Autodesk Fusion 360 part; units mm, degrees
sketch "Sketch1" plane through (0, 0, 0) normal (0, 0, 1) x (1, 0, 0)
  line L0 (2.6252, 0) -> (7.4595, 0)
  line L1 (10.0424, 2.5828) -> (10.0424, 3.3)
  line L2 (0.0424, 3.3) -> (0.0424, 2.5828)
  line L3 (8.0424, 3.7) -> (8.0424, 4.8)
  line L4 (2.0424, 4.8) -> (2.0424, 3.7)
  line L5 (0.101, 2.4414) -> (2.4838, 0.0586)
  line L6 (0.0424, 2.5) -> (3.5052, 2.5) construction
  line L7 (5.0424, 3.5) -> (5.0424, 0) construction
  line L8 (9.9838, 2.4414) -> (7.601, 0.0586)
  line L9 (9.8424, 3.5) -> (8.2424, 3.5)
  line L10 (1.8424, 3.5) -> (0.2424, 3.5)
  line L11 (5.0424, 4.7) -> (5.3424, 5)
  line L12 (5.0424, 4.7) -> (6.213, 4.7) construction
  line L13 (5.0424, 4.7) -> (4.7424, 5)
  line L14 (5.0424, 4.7) -> (6.2088, 4.7) construction
  line L15 (7.8424, 5) -> (5.3424, 5)
  line L16 (4.7424, 5) -> (2.2424, 5)
  arc A0 (0.2424, 3.5) -> (0.0424, 3.3) centre (0.2424, 3.3) ccw
  arc A1 (0.0424, 2.5828) -> (0.101, 2.4414) centre (0.2424, 2.5828) ccw
  arc A2 (2.4838, 0.0586) -> (2.6252, 0) centre (2.6252, 0.2) ccw
  arc A3 (7.4595, 0) -> (7.601, 0.0586) centre (7.4595, 0.2) ccw
  arc A4 (9.9838, 2.4414) -> (10.0424, 2.5828) centre (9.8424, 2.5828) ccw
  arc A5 (10.0424, 3.3) -> (9.8424, 3.5) centre (9.8424, 3.3) ccw
  arc A6 (8.0424, 3.7) -> (8.2424, 3.5) centre (8.2424, 3.7) ccw
  arc A7 (8.0424, 4.8) -> (7.8424, 5) centre (7.8424, 4.8) ccw
  arc A8 (2.2424, 5) -> (2.0424, 4.8) centre (2.2424, 4.8) ccw
  arc A9 (1.8424, 3.5) -> (2.0424, 3.7) centre (1.8424, 3.7) ccw
  dimension "d1" = 10
  dimension "d4" = 5
  dimension "d5" = 45
  dimension "d6" = 1
  dimension "d7" = 5
  dimension "d8" = 6
  dimension "d9" = 2
  dimension "d10" = 2
  dimension "d12" = 45
  dimension "d13" = 0.3
  dimension "d14" = 5
  dimension "d15" = 1.5
  dimension "d16" = 0.2
extrude "Extrude1" add sketch "Sketch1" along normal blind 10
hole "Hole1" at (5.0424, 5, 5) direction (0, -1, 0) diameter 4.234 depth 5.834 tip angle 180 countersink diameter 6 countersink angle 90
Build history of the part. All positions in model axes, mm. A direction names the side the tool comes from. Coordinates: 2 decimals unless noted, no trailing zeros. Order: outer loops, then holes, each group sorted by start corner. A loop starts at its lowest first (then second) coordinate and runs counter-clockwise, first axis right, second up. Notation, with made-up numbers: M 69.5,36 L 117.5,36 A15 ccw 117.5,49 Z; hole C -37.75,76.5 d8. An arc over 180 degrees is marked long. One line per question, with ' | ' between items. Start each with the question number.
1. Tool access for faces 5 (the face through (7, 5, 1)), 6 (the face through (1, 3.5, 5)), 7 (the face through (8.042, 4, 5)): list every direction of +Z, -Z, +X, -X, +Y, -Y with a clear straight run to the whole face (end or side of a thin tool).
2. Flat gauge pins, fed straight in: P1, Ø1, axis at x = 5, z = 6.5, coming from the +Y side; P2, Ø1.3, axis at x = 1, z = 4.5, coming from the +Y side; P3, Ø0.5, axis at y = 4, z = 4, coming from the -X side; P4, Ø6, axis at x = 2, z = 1.5, coming from the -Y side. Where does each tip first touch, or does it go through?
3. Cut at A-A (z = 5). Write the cut outline in (x, y), plus the area to 3 significant figures.
4. Wall check: line 1 along Y through (x, z) = (5, 9.5); line 2 along Y through (x, z) = (7, 7); line 3 along X through (y, z) = (3.3, 6.5). Give the ranges that are in metal, low to high. Write a range as [from, to].
5. Cut at B-B (y = 0.5). Write the cut outline in (x, z), plus the area to 3 significant figures.
6. Cut at C-C (z = 8.5). Write the cut outline in (x, y).
7. Cut at D-D (y = 4.25). Write the cut outline in (x, z), plus the area to 3 significant figures.
8. Mould opens along Z. For faces 1 (the face through (7.1, 2, 4.5)), 2 (the face through (4, 5, 1)), 3 (the face through (5, 3, 0)), 4 (the face through (5, 3, 10)) say: +Z half, -Z half, draft (parallel to the pull), parting line (faces both ways), or undercut.
The answers:
1) face 5: +Z, -Z, +X, -X, +Y | face 6: +Z, -Z, -X, +Y | face 7: +Z, -Z, +X, +Y
2) P1: passes through | P2: stops at y = 3.5 | P3: stops at x = 2.04 | P4: stops at y = 0
3) outline: M 0.04,2.58 A0.2 ccw 0.1,2.44 L 2.48,0.06 A0.2 ccw 2.63,0 L 2.93,0 L 2.93,4.12 L 2.1,4.94 A0.2 ccw 2.04,4.8 L 2.04,3.7 A0.2 cw 1.84,3.5 L 0.24,3.5 A0.2 ccw 0.04,3.3 Z; M 7.16,0 L 7.46,0 A0.2 ccw 7.6,0.06 L 9.98,2.44 A0.2 ccw 10.04,2.58 L 10.04,3.3 A0.2 ccw 9.84,3.5 L 8.24,3.5 A0.2 cw 8.04,3.7 L 8.04,4.8 A0.2 ccw 7.98,4.94 L 7.16,4.12 Z | area: 15.8 mm2
4) line 1: y = [0, 4.74] | line 2: y = [0, 4.8] | line 3: x = [0.04, 3.55], [6.54, 10.04]
5) outline: M 2.04,0 L 8.04,0 L 8.04,10 L 2.04,10 Z; hole C 5.04,5 d4.23 | area: 45.9 mm2
6) outline: M 0.04,2.58 A0.2 ccw 0.1,2.44 L 2.48,0.06 A0.2 ccw 2.63,0 L 7.46,0 A0.2 ccw 7.6,0.06 L 9.98,2.44 A0.2 ccw 10.04,2.58 L 10.04,3.3 A0.2 ccw 9.84,3.5 L 8.24,3.5 A0.2 cw 8.04,3.7 L 8.04,4.8 A0.2 ccw 7.84,5 L 5.34,5 L 5.04,4.7 L 4.74,5 L 2.24,5 A0.2 ccw 2.04,4.8 L 2.04,3.7 A0.2 cw 1.84,3.5 L 0.24,3.5 A0.2 ccw 0.04,3.3 Z
7) outline: M 2.04,0 L 8.04,0 L 8.04,10 L 2.04,10 Z; hole C 5.04,5 d4.5 | area: 44.1 mm2
8) face 1: undercut | face 2: draft | face 3: -Z half | face 4: +Z half
